Verification items for the finished model (mm, model axes). A direction names the side the tool comes from. Give positions to 0.01 mm unless a question says otherwise; leave off trailing zeros. Order: outer loops, then holes, each group sorted by start corner. A loop starts at its lowest first (then second) coordinate and runs counter-clockwise, first axis right, second up. Notation, with made-up numbers: (83.5, -21.5) -> (109.5, -21.5) arc R11 cw to (109.5, -0.5) -> close; hole circle Ø4 at (88, 16). An arc over 180 degrees is marked (long way). Return JSON: item names as keys, results as strings. Group by question number.
(1) Depth check by flat-ended pin: pin 1 Ø2 at (y, z) = (16.5, 4) entering from -X; pin 2 Ø8 at (x, y) = (15, 29.5) entering from +Z; pin 3 Ø1.5 at (x, y) = (16, 11) entering from +Z; pin 4 Ø5 at (y, z) = (-3.5, 1) entering from -X. Enter the tip coordinate at first touch or a pass-through.
(2) Tool access check on faces 1 (the face through (-4.93, -1.773, -0.379)), 2 (the face through (-10, 0, 0)). Record the directions out of +Z, -Z, +X, -X, +Y, -Y that give a thin tool (end or side, any length) a straight path to the whole face; none if there is none.
(3) Cross-section at A-A on z = 0. Enter the section's corners in (x, y).
(4) Thickness scan on line 1 along X through (y, z) = (17, -1.5); line 2 along Y through (x, z) = (24, -0.5); line 3 along Z through (x, y) = (19, 29.5). Record the ranges inside material, lowest first.
from build123d import *

# Parameters (mm, degrees)
SALIENTE_EXTRUIR1_DEPTH    = 37.5
CORTAR_EXTRUIR1_DEPTH      = 37.5
CORTAR_EXTRUIR1_DEPTH_BACK = 37.5
CROQUIS3_R                 = 1.75
SALIENTE_EXTRUIR2_DEPTH    = 10
REDONDEO1_R                = 0.75


with BuildPart() as part:
    # Croquis1 → Saliente-Extruir1 (new body)
    with BuildSketch(Plane(origin=(0, 0, 0), x_dir=(0, 0, -1), z_dir=(1, 0, 0))):
        Polygon((-6, -8.564759036), (6, -8.564759036), (1.75, 37.935240964), (-1.75, 37.935240964), align=None)
    extrude(amount=SALIENTE_EXTRUIR1_DEPTH)

    # Croquis2 → Cortar-Extruir1 (cut, two sides: drawn at the far end of the back side and taken through both)
    with BuildSketch(Plane.XY.offset(-CORTAR_EXTRUIR1_DEPTH_BACK)):
        Polygon((0, 37.935240964), (37.5, 37.935240964), (37.5, 34.654416082), align=None)
    extrude(amount=CORTAR_EXTRUIR1_DEPTH + CORTAR_EXTRUIR1_DEPTH_BACK, mode=Mode.SUBTRACT)

    # Croquis3 → Saliente-Extruir2 (add)
    with BuildSketch(Plane.ZY):
        with Locations((0, -0.064759036)):
            Circle(CROQUIS3_R)
    extrude(amount=SALIENTE_EXTRUIR2_DEPTH)

    # Redondeo1
    redondeo1_edges = [part.edges().sort_by_distance(p)[0] for p in [
        (37.5, 13.044828523, 4.024930169),
        (37.5, 34.654416082, 0),
        (37.5, -8.564759036, 0),
        (18.75, 36.294828523, -1.899930169),
        (18.75, 36.294828523, 1.899930169),
        (37.5, 13.044828523, -4.024930169),
        (0, -8.564759036, 0),
        (0, 14.685240964, 3.875),
        (0, 37.935240964, 0),
        (0, 14.685240964, -3.875),
        (18.75, -8.564759036, -6),
        (18.75, -8.564759036, 6),
    ]]
    fillet(redondeo1_edges, radius=REDONDEO1_R)


solid = part.part
Verdict:
{
 "1": {"pin 1": "x = 0", "pin 2": "z = 2.89", "pin 3": "z = 4.28", "pin 4": "x = -10"},
 "2": {"face 1": "-X", "face 2": "+Z, -Z, -X, +Y, -Y"},
 "3": {"outline": "(-10, -1.81) -> (0, -1.81) -> (0, -7.81) arc R0.75 ccw to (0.75, -8.56) -> (36.75, -8.56) arc R0.75 ccw to (37.5, -7.81) -> (37.5, 33.97) arc R0.75 ccw to (36.82, 34.71) -> (0.82, 37.86) arc R0.75 ccw to (0, 37.12) -> (0, 1.69) -> (-10, 1.69) -> close"},
 "4": {"line 1": "0 to 37.5", "line 2": "-8.56 to 35.84", "line 3": "-2.52 to 2.52"}
}
